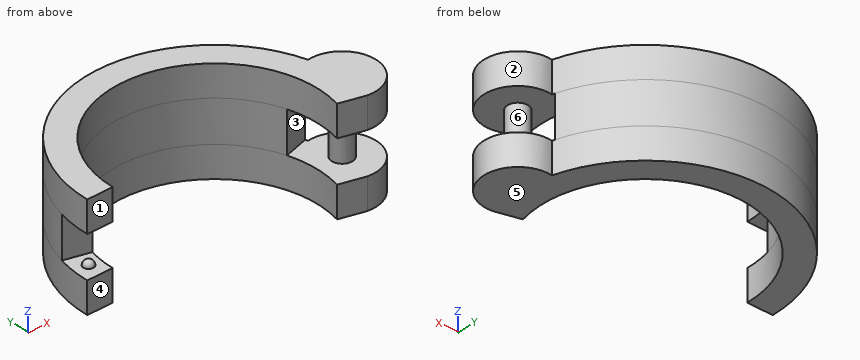
from build123d import *

# Parameters (mm, degrees)
F1_DEPTH = 3
F2_R     = 1
F3_DEPTH = 4
F5_DEPTH = 3


with BuildPart() as f1:
    # F0 (on Top) → F1 (new body)
    with BuildSketch(Plane.XY):
        with BuildLine():
            Line((9.6592582629, -2.588190451), (12.0740728286, -3.2352380638))
            ThreePointArc((12.0740728286, -3.2352380638), (12.5, 0), (12.0740728286, 3.2352380638))
            ThreePointArc((12.0740728286, 3.2352380638), (-1.6315774028, 12.3930607672), (-12.5, 0))
            Line((-12.5, 0), (-10, 0))
            ThreePointArc((-10, 0), (1.3052619222, 9.9144486137), (9.6592582629, -2.588190451))
        make_face()
        with BuildLine():
            ThreePointArc((12.0740728286, 3.2352380638), (12.5, 0), (12.0740728286, -3.2352380638))
            ThreePointArc((12.0740728286, -3.2352380638), (15.7631548055, 0), (12.0740728286, 3.2352380638))
        make_face()
    extrude(amount=F1_DEPTH)

    # F2 (on face) → F3 (join)
    with BuildSketch(Plane.XY.offset(3)):
        with Locations((12.5, 0)):
            Circle(F2_R)
        with BuildLine():
            Line((-12.0740728286, 3.2352380638), (-9.6592582629, 2.588190451))
            ThreePointArc((-9.6592582629, 2.588190451), (-0.100929954, 9.9994906442), (9.605047786, 2.7826349075))
            Line((9.605047786, 2.7826349075), (12.0063097325, 3.4782936344))
            ThreePointArc((12.0063097325, 3.4782936344), (-0.1261624425, 12.4993633053), (-12.0740728286, 3.2352380638))
        make_face()
    extrude(amount=F3_DEPTH)

    # F4 (on face) → F5 (join)
    with BuildSketch(Plane.XY.offset(7)):
        with BuildLine():
            Line((9.6592582629, -2.588190451), (12.0740728286, -3.2352380638))
            ThreePointArc((12.0740728286, -3.2352380638), (12.5, 0), (12.0740728286, 3.2352380638))
            ThreePointArc((12.0740728286, 3.2352380638), (-1.6315774028, 12.3930607672), (-12.5, 0))
            Line((-12.5, 0), (-10, 0))
            ThreePointArc((-10, 0), (1.3052619222, 9.9144486137), (9.6592582629, -2.588190451))
        make_face()
        with BuildLine():
            ThreePointArc((12.0740728286, 3.2352380638), (12.5, 0), (12.0740728286, -3.2352380638))
            ThreePointArc((12.0740728286, -3.2352380638), (15.7631548055, 0), (12.0740728286, 3.2352380638))
        make_face()
    extrude(amount=F5_DEPTH)

    # F6 (on face) → F7 (revolve)
    with BuildSketch(Plane.XY.offset(3)):
        with BuildLine():
            Line((-11.123595869, 0.960134698), (-10.9930696768, 1.9515795594))
            ThreePointArc((-10.9930696768, 1.9515795594), (-11.5540552036, 1.5211202248), (-11.123595869, 0.960134698))
        make_face()
    revolve(axis=Axis((-11.0583327729, 1.4558571287, 3), (-0.1305261922, -0.9914448614, 0)))


solid = f1.part
For this review, take the finished solid that the model builds, in its own axes (mm). Face numbers are marked on the shaded views. A direction names the side the tool comes from. Round coordinates to 2 decimals unless told otherwise and drop trailing zeros. Loops run counter-clockwise (first coordinate to the right, second up) from the corner with the lowest first, then second, coordinate; pieces in that order, holes last. Notation, with made-up numbers: (38, 74.5) - (94, 74.5) arc R23 ccw to (94, 90.5) - close; hole circle Ø2 at (-37, 43.25). An arc over 180 degrees is marked (long way). Use one line per item in the form item = value.
1) Clearance check with flat-ended pins moving along their axes: P1, Ø8, axis at x = 3, y = 2.5, coming from the -Z side; P2, Ø1, axis at x = -1, z = 5, coming from the +Y side; P3, Ø5, axis at y = 9.5, z = 8, coming from the +X side; P4, Ø1.5, axis at x = 5.5, z = 6, coming from the -Y side. State where each tip first meets the part, or that it passes through.
Solutions:
P1 = through
P2 = 12.49
P3 = 10.36
P4 = 7.81
2) Mouldability with a two-part tool opening along Y and no side actions: class the marked faces 1, 2 and 3 as pulls with the +Y half, pulls with the -Y half, needs draft (parallel to the pull), parting line crosses it, or undercut.
Solutions:
face_1 = pulls with the -Y half
face_2 = parting line crosses it
face_3 = undercut
3) We need section D-D on y = 1.5. Write out the cut boundary in (x, z).
Solutions:
outline = (-12.41, 0) - (-9.89, 0) - (-9.89, 3) - (-10.56, 3) arc R0.5 ccw to (-11.56, 3) - (-12.41, 3) - close; (-12.41, 7) - (-9.89, 7) - (-9.89, 10) - (-12.41, 10) - close; (9.89, 0) - (15.4, 0) - (15.4, 3) - (9.89, 3) - close; (9.89, 7) - (15.4, 7) - (15.4, 10) - (9.89, 10) - close
4) We need section A-A on y = 4.5. Write out the cut boundary in (x, z).
Solutions:
outline = (-11.66, 0) - (-8.93, 0) - (-8.93, 10) - (-11.66, 10) - close; (8.93, 0) - (11.66, 0) - (11.66, 10) - (8.93, 10) - close
5) Wall thickness on probe 1 along Z at (x, y) = (12.25, -1.5); probe 2 along X at (y, z) = (5, 1); probe 3 along Y at (x, z) = (0, 1.2): over which ranges is each line inside the solid? List them lowest first.
Solutions:
probe_1 = 0 to 3, 7 to 10
probe_2 = -11.46 to -8.66, 8.66 to 11.46
probe_3 = 10 to 12.5
6) We need section B-B on x = 12.5. Write out the cut boundary in (y, z).
Solutions:
outline = (-3.26, 0) - (3.26, 0) - (3.26, 3) - (1, 3) - (1, 7) - (3.26, 7) - (3.26, 10) - (-3.26, 10) - (-3.26, 7) - (-1, 7) - (-1, 3) - (-3.26, 3) - close
7) We need section C-C on z = 1. Write out the cut boundary in (x, y).
Solutions:
outline = (-12.5, 0) - (-10, 0) arc R10 cw (long way) to (9.66, -2.59) - (12.07, -3.24) arc R3.26 ccw (long way) to (12.07, 3.24) arc R12.5 ccw to start
8) Tool access review of the marked faces 4, 5 and 6: name each direction out of +Z, -Z, +X, -X, +Y, -Y from which nothing blocks a thin tool from reaching the whole face with its end or side.
Solutions:
face_4 = +Z, -Z, -X, -Y
face_5 = -Z, +X, -X, +Y, -Y
face_6 = none
